```python
from build123d import *

# Parameters (mm, degrees)
SKETCH1_R           = 1
SKETCH1_R_2         = 1.4
SKETCH1_R_3         = 3
SKETCH1_RX          = 16.5
SKETCH1_RY          = 8
BOSS_EXTRUDE1_DEPTH = 5
CUT_EXTRUDE1_REACH  = 153.803
SKETCH2_R           = 3.875


with BuildPart() as part:
    # Sketch1 → Boss-Extrude1 (new body)
    with BuildSketch(Plane.XY):
        with BuildLine():
            Line((-14, 0), (-14, 44.641437436))
            ThreePointArc((-14, 44.641437436), (-13.783259018, 45.164696454), (-13.26, 45.381437436))
            Line((-13.26, 45.381437436), (-13.24, 45.381437436))
            ThreePointArc((-13.24, 45.381437436), (-12.716740982, 45.598178417), (-12.5, 46.121437436))
            Line((-12.5, 46.121437436), (-12.5, 56.641437436))
            ThreePointArc((-12.5, 56.641437436), (-12.716740982, 57.164696454), (-13.24, 57.381437436))
            Line((-13.24, 57.381437436), (-13.26, 57.381437436))
            ThreePointArc((-13.26, 57.381437436), (-13.783259018, 57.598178417), (-14, 58.121437436))
            Line((-14, 58.121437436), (-14, 135.347392982))
            ThreePointArc((-14, 135.347392982), (-13.809166738, 136.199986504), (-13.273084285, 136.889876824))
            ThreePointArc((-13.273084285, 136.889876824), (-11.805402668, 140.00423401), (-13.273084285, 143.118591196))
            ThreePointArc((-13.273084285, 143.118591196), (-13.809166738, 143.808481515), (-14, 144.661075038))
            Line((-14, 144.661075038), (-14, 149.07320666))
            ThreePointArc((-14, 149.07320666), (-13.162476387, 150.700673602), (-11.351351351, 150.965098552))
            ThreePointArc((-11.351351351, 150.965098552), (0, 149.07320666), (11.351351351, 150.965098552))
            ThreePointArc((11.351351351, 150.965098552), (13.162476387, 150.700673602), (14, 149.07320666))
            Line((14, 149.07320666), (14, 144.661075038))
            ThreePointArc((14, 144.661075038), (13.809166738, 143.808481515), (13.273084285, 143.118591196))
            ThreePointArc((13.273084285, 143.118591196), (11.805402668, 140.00423401), (13.273084285, 136.889876824))
            ThreePointArc((13.273084285, 136.889876824), (13.809166738, 136.199986504), (14, 135.347392982))
            Line((14, 135.347392982), (14, 58.121437436))
            ThreePointArc((14, 58.121437436), (13.783259018, 57.598178417), (13.26, 57.381437436))
            Line((13.26, 57.381437436), (13.24, 57.381437436))
            ThreePointArc((13.24, 57.381437436), (12.716740982, 57.164696454), (12.5, 56.641437436))
            Line((12.5, 56.641437436), (12.5, 46.121437436))
            ThreePointArc((12.5, 46.121437436), (12.716740982, 45.598178417), (13.24, 45.381437436))
            Line((13.24, 45.381437436), (13.26, 45.381437436))
            ThreePointArc((13.26, 45.381437436), (13.783259018, 45.164696454), (14, 44.641437436))
            Line((14, 44.641437436), (14, 0))
            ThreePointArc((14, 0), (0, -14), (-14, 0))
        make_face()
        with Locations((-8, 144.371191598)):
            Circle(SKETCH1_R, mode=Mode.SUBTRACT)
        with Locations((6.717514421, -6.717514421)):
            Circle(SKETCH1_R_2, mode=Mode.SUBTRACT)
        with Locations((-5.656854249, -5.656854249)):
            Circle(SKETCH1_R_2, mode=Mode.SUBTRACT)
        with Locations(Location((5.656854249, 5.656854249, 0), (0, 0, 180))):
            Circle(SKETCH1_R_2, mode=Mode.SUBTRACT)
        with Locations(Location((-6.717514421, 6.717514421, 0), (0, 0, 180))):
            Circle(SKETCH1_R_2, mode=Mode.SUBTRACT)
        with Locations(Location((8, 144.371191598, 0), (0, 0, 180))):
            Circle(SKETCH1_R, mode=Mode.SUBTRACT)
        with Locations((0, 136.07320666)):
            Circle(SKETCH1_R, mode=Mode.SUBTRACT)
        with Locations((7.903282752, 93.738271437)):
            Circle(SKETCH1_R, mode=Mode.SUBTRACT)
        with Locations((8.715574275, 84.453736851)):
            Circle(SKETCH1_R_3, mode=Mode.SUBTRACT)
        with Locations(Location((-7.903282752, 93.738271437, 0), (0, 0, 180))):
            Circle(SKETCH1_R, mode=Mode.SUBTRACT)
        with Locations(Location((-8.715574275, 84.453736851, 0), (0, 0, 180))):
            Circle(SKETCH1_R_3, mode=Mode.SUBTRACT)
        with Locations(Location((0, 111.383897204), (0, 0, 90))):
            Ellipse(SKETCH1_RX, SKETCH1_RY, mode=Mode.SUBTRACT)
        with BuildLine():
            Line((-4, 29.983897204), (4, 29.983897204))
            ThreePointArc((4, 29.983897204), (5.414213562, 30.569683642), (6, 31.983897204))
            Line((6, 31.983897204), (6, 32.983897204))
            ThreePointArc((6, 32.983897204), (5.414213562, 34.398110767), (4, 34.983897204))
            Line((4, 34.983897204), (-4, 34.983897204))
            ThreePointArc((-4, 34.983897204), (-5.414213562, 34.398110767), (-6, 32.983897204))
            Line((-6, 32.983897204), (-6, 31.983897204))
            ThreePointArc((-6, 31.983897204), (-5.414213562, 30.569683642), (-4, 29.983897204))
        make_face(mode=Mode.SUBTRACT)
        with BuildLine():
            Line((-4, 20.483897204), (4, 20.483897204))
            ThreePointArc((4, 20.483897204), (5.414213562, 21.069683642), (6, 22.483897204))
            Line((6, 22.483897204), (6, 23.483897204))
            ThreePointArc((6, 23.483897204), (5.414213562, 24.898110767), (4, 25.483897204))
            Line((4, 25.483897204), (-4, 25.483897204))
            ThreePointArc((-4, 25.483897204), (-5.414213562, 24.898110767), (-6, 23.483897204))
            Line((-6, 23.483897204), (-6, 22.483897204))
            ThreePointArc((-6, 22.483897204), (-5.414213562, 21.069683642), (-4, 20.483897204))
        make_face(mode=Mode.SUBTRACT)
        with BuildLine():
            Line((-3.5, 42.443937436), (3.5, 42.443937436))
            ThreePointArc((3.5, 42.443937436), (4.207106781, 42.736830654), (4.5, 43.443937436))
            Line((4.5, 43.443937436), (4.5, 76.443937436))
            ThreePointArc((4.5, 76.443937436), (4.207106781, 77.151044217), (3.5, 77.443937436))
            Line((3.5, 77.443937436), (-3.5, 77.443937436))
            ThreePointArc((-3.5, 77.443937436), (-4.207106781, 77.151044217), (-4.5, 76.443937436))
            Line((-4.5, 76.443937436), (-4.5, 43.443937436))
            ThreePointArc((-4.5, 43.443937436), (-4.207106781, 42.736830654), (-3.5, 42.443937436))
        make_face(mode=Mode.SUBTRACT)
    extrude(amount=BOSS_EXTRUDE1_DEPTH)

    # Sketch2 → Cut-Extrude1 (cut, up to next)
    with BuildSketch(Plane.XY.offset(5), mode=Mode.PRIVATE) as cut_extrude1_sk1:
        Circle(SKETCH2_R)
    cut_extrude1_tool1 = extrude(cut_extrude1_sk1.sketch, amount=-CUT_EXTRUDE1_REACH, mode=Mode.PRIVATE) & part.part
    add(cut_extrude1_tool1.solids().sort_by_distance((0, 0, 5))[0], mode=Mode.SUBTRACT)


solid = part.part
```
Part model, mm, in its own coordinate system. A direction names the side the tool comes from. Round coordinates to 2 decimals unless told otherwise and drop trailing zeros.
Item 1: Cut at A-A, the plane z = 3.7. State how many separate pieces and enclosed holes the cut face has, then the cut area to 3 significant figures.
Item 2: 3-axis set-ups, long thin cutter, end or side, ignore diameter. For faces 1 (the face through (-14, 96, 2)), 2 (the face through (-12.5, 51, 2)), 3 (the face through (0, 29.984, 2)): which of +Z, -Z, +X, -X, +Y, -Y reach the whole face in a straight line?
Item 3: Drill centre lines: line 1 (X direction, y = 25, z = 3); line 2 (X direction, y = 86, z = 0.5); line 3 (X direction, y = 46.5, z = 0.85). Where is each one in solid material? Low to high.
Item 4: Drop flat-ended pins along their axis: P1, Ø7, axis at x = 0, y = 0, coming from the -Z side; P2, Ø1.5, axis at x = 5.5, z = 2.5, coming from the +Y side; P3, Ø3, axis at x = -9.5, z = 3.5, coming from the -Y side; P4, Ø2.5, axis at x = 0.5, z = 2, coming from the +Y side. Give the stop position or say it passes through.
Item 5: Mould opens along X. For faces 4 (the face through (14, 23, 2)), 5 (the face through (0, 20.484, 2)), 6 (the face through (-11.806, 139.954, 2.465)) say: +X half, -X half, draft (parallel to the pull), parting line (faces both ways), or undercut.
A:
1. separate pieces: 1
1. enclosed holes: 16
1. area: 3,460 mm2
2. face 1: +Z, -Z, -X, +Y, -Y
2. face 2: +Z, -Z, -X
2. face 3: +Z, -Z
3. line 1: x = -14 to -5.3, 5.3 to 14
3. line 2: x = -14 to -11.29, -6.14 to 6.14, 11.29 to 14
3. line 3: x = -12.5 to -4.5, 4.5 to 12.5
4. P1: passes through
4. P2: stops at y = 149.64
4. P3: stops at y = -11.49
4. P4: stops at y = 149.12
5. face 4: +X half
5. face 5: undercut
5. face 6: -X half
